Input: part model. Units: mm. Frame: model coordinates. Round coordinates to 2 decimals unless told otherwise and drop trailing zeros. Loops run counter-clockwise (first coordinate to the right, second up) from the corner with the lowest first, then second, coordinate; pieces in that order, holes last.
1) Ray query, line 1 along X through (y, z) = (-0.3, 0). Return the intervals inside material, ascending.
2) Section B-B, the plane z = -0.5. Return loops of the section in (x, y), and give its area (3 significant figures).
3) Section A-A, the plane y = 0.1. Return loops of the section in (x, z), and give its area (3 significant figures).
4) First-contact query: pin 1 (2.5 mm diameter, centred on y = -0.5, z = 0.5, fed in from +X); pin 2 (2.5 mm diameter, centred on y = -1, z = 1, fed in from -X). Flat tips, straight axial feed; report the tip coordinate or a pass-through.
from build123d import *

# Parameters (mm, degrees)
PAD_DEPTH = 2.5


with BuildPart() as part:
    # Sketch → Pad (new body, symmetric)
    with BuildSketch(Plane.XZ):
        Polygon((0, 7.5), (0, 2.55), (10, 2.55), (10, -2.55), (0, -2.55), (0, -7.5), (240, -7.5), (240, -2.55), (230, -2.55), (230, 2.55), (240, 2.55), (240, 7.5), align=None)
    extrude(amount=PAD_DEPTH, both=True)


solid = part.part
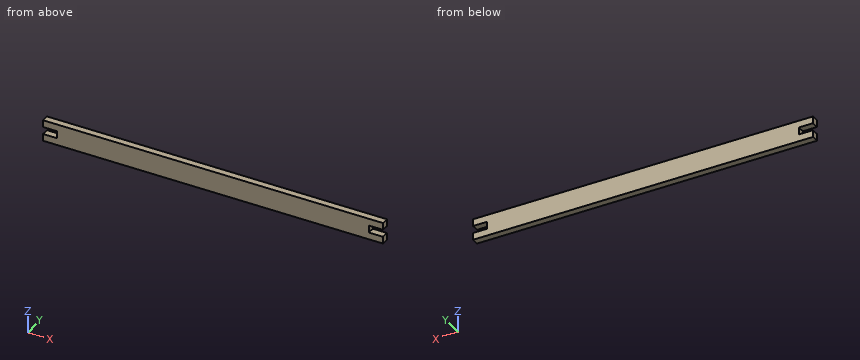
Final values:
1. line 1: x = 10 to 230
2. outline: (10, -2.5) - (230, -2.5) - (230, 2.5) - (10, 2.5) - close
2. area: 1,100 mm2
3. outline: (0, -7.5) - (240, -7.5) - (240, -2.55) - (230, -2.55) - (230, 2.55) - (240, 2.55) - (240, 7.5) - (0, 7.5) - (0, 2.55) - (10, 2.55) - (10, -2.55) - (0, -2.55) - close
3. area: 3,500 mm2
4. pin 1: stops at x = 230
4. pin 2: stops at x = 10
